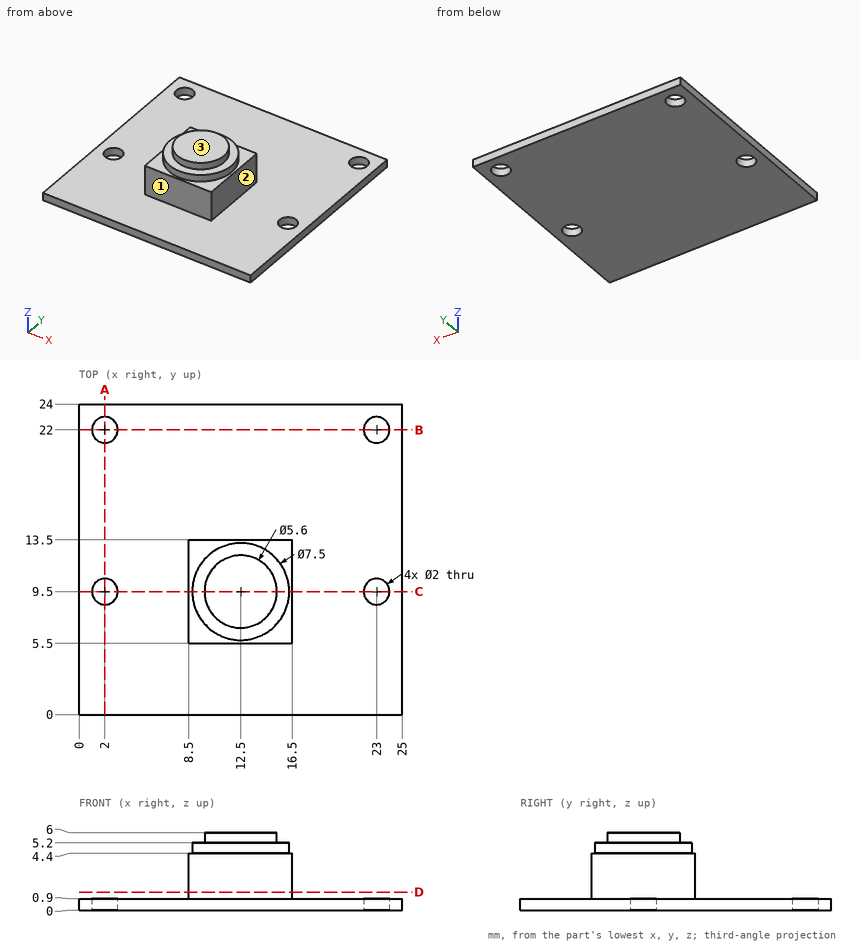
Part print with two shaded views. Sizes in mm from the minimum x, y, z corner. A direction names the side the tool comes from. Round coordinates to 2 decimals unless told otherwise and drop trailing zeros. Order: outer loops, then holes, each group sorted by start corner. A loop starts at its lowest first (then second) coordinate and runs counter-clockwise, first axis right, second up.
(1) Band-saw the part on A-A (x = 2). List the corners of the cut face in (y, z).
(2) Pin check, flat tips, straight feed: pin 1 (4 mm diameter, centred on x = 21, y = 21, fed in from -Z); pin 2 (3 mm diameter, centred on y = 9, z = 2.5, fed in from -X); pin 3 (6 mm diameter, centred on x = 10, y = 21, fed in from +Z); pin 4 (1 mm diameter, centred on x = 11, z = 3, fed in from -Y). Stop position of each tip, or through.
(3) Drill centre lines: line 1 (Y direction, x = 2, z = 0.5); line 2 (Z direction, x = 15.25, y = 17.75); line 3 (X direction, y = 10, z = 1.95). Where is each one in solid material? Low to high.
(4) 3-axis set-ups, long thin cutter, end or side, ignore diameter. For the marked faces 1, 2 and 3: which of +Z, -Z, +X, -X, +Y, -Y reach the whole face in a straight line?
(5) Band-saw the part on D-D (z = 1.4). List the corners of the cut face in (x, y), then the cut area to 3 significant figures.
(6) Band-saw the part on B-B (y = 22). List the corners of the cut face in (x, z), then the cut area to 3 significant figures.
(7) Band-saw the part on C-C (y = 9.5). List the corners of the cut face in (x, z), then the cut area to 3 significant figures.
Verdict:
1. outline: (0, 0) - (8.5, 0) - (8.5, 0.9) - (0, 0.9) - close; (10.5, 0) - (21, 0) - (21, 0.9) - (10.5, 0.9) - close; (23, 0) - (24, 0) - (24, 0.9) - (23, 0.9) - close
2. pin 1: stops at z = 0
2. pin 2: stops at x = 8.5
2. pin 3: stops at z = 0.9
2. pin 4: stops at y = 5.5
3. line 1: y = 0 to 8.5, 10.5 to 21, 23 to 24
3. line 2: z = 0 to 0.9
3. line 3: x = 8.5 to 16.5
4. face 1: +Z, +X, -X, -Y
4. face 2: +Z, +X, +Y, -Y
4. face 3: +Z, +X, -X, +Y, -Y
5. outline: (8.5, 5.5) - (16.5, 5.5) - (16.5, 13.5) - (8.5, 13.5) - close
5. area: 64.0 mm2
6. outline: (0, 0) - (1, 0) - (1, 0.9) - (0, 0.9) - close; (3, 0) - (22, 0) - (22, 0.9) - (3, 0.9) - close; (24, 0) - (25, 0) - (25, 0.9) - (24, 0.9) - close
6. area: 18.9 mm2
7. outline: (0, 0) - (1, 0) - (1, 0.9) - (0, 0.9) - close; (3, 0) - (22, 0) - (22, 0.9) - (16.5, 0.9) - (16.5, 4.4) - (16.25, 4.4) - (16.25, 5.2) - (15.3, 5.2) - (15.3, 6) - (9.7, 6) - (9.7, 5.2) - (8.75, 5.2) - (8.75, 4.4) - (8.5, 4.4) - (8.5, 0.9) - (3, 0.9) - close; (24, 0) - (25, 0) - (25, 0.9) - (24, 0.9) - close
7. area: 57.4 mm2
